```python
from build123d import *

# Parameters (mm, degrees)
SKETCH1_W           = 80
SKETCH1_H           = 100
BOSS_EXTRUDE1_DEPTH = 5
SKETCH2_W           = 80
SKETCH2_H           = 5
BOSS_EXTRUDE2_DEPTH = 20
SKETCH3_R           = 4
CUT_EXTRUDE1_DEPTH  = 107.066017178
SKETCH4_R           = 4
CUT_EXTRUDE2_DEPTH  = 68.082039325
SKETCH5_R           = 3
CUT_EXTRUDE4_DEPTH  = 68.082039325
SKETCH7_R           = 3
CUT_EXTRUDE5_DEPTH  = 10


with BuildPart() as part:
    # Sketch1 → Boss-Extrude1 (new body)
    with BuildSketch(Plane(origin=(0, 0, 0), x_dir=(0, 0, -1), z_dir=(1, 0, 0))):
        Rectangle(SKETCH1_W, SKETCH1_H)
    extrude(amount=BOSS_EXTRUDE1_DEPTH)

    # Sketch2 → Boss-Extrude2 (add)
    with BuildSketch(Plane(origin=(5, 0, 0), x_dir=(0, 0, -1), z_dir=(1, 0, 0))):
        with Locations((0, -47.5)):
            Rectangle(SKETCH2_W, SKETCH2_H)
    extrude(amount=BOSS_EXTRUDE2_DEPTH)

    # Sketch3 → Cut-Extrude1 (cut, through all)
    with BuildSketch(Plane(origin=(0, -45, 0), x_dir=(1, 0, 0), z_dir=(0, 1, 0))):
        with Locations(Location((14, 25, 0), (0, 0, 270))):
            Circle(SKETCH3_R)
        with Locations(Location((14, -25, 0), (0, 0, 270))):
            Circle(SKETCH3_R)
    extrude(amount=-CUT_EXTRUDE1_DEPTH, mode=Mode.SUBTRACT)

    # Sketch4 → Cut-Extrude2 (cut, through all)
    with BuildSketch(Plane(origin=(5, 0, 0), x_dir=(0, 0, -1), z_dir=(1, 0, 0))):
        with Locations((3, -18)):
            Circle(SKETCH4_R)
    extrude(amount=-CUT_EXTRUDE2_DEPTH, mode=Mode.SUBTRACT)

    # Sketch5 → Cut-Extrude4 (cut, through all)
    with BuildSketch(Plane(origin=(5, 0, 0), x_dir=(0, 0, -1), z_dir=(1, 0, 0))):
        with BuildLine():
            Line((-40, 50), (-40, 0))
            ThreePointArc((-40, 0), (-36.772544511, 5.320995859), (-30.562334356, 4.917565955))
            ThreePointArc((-30.562334356, 4.917565955), (-15.830972977, -2.382340063), (0.39983188, -5.001998369))
            ThreePointArc((0.39983188, -5.001998369), (28.425281663, -16.857445702), (40, -45))
            Line((40, -45), (40, 50))
            Line((40, 50), (-40, 50))
        make_face()
        with Locations((-34, 0)):
            Circle(SKETCH5_R)
    extrude(amount=-CUT_EXTRUDE4_DEPTH, mode=Mode.SUBTRACT)

    # Sketch7 → Cut-Extrude5 (cut)
    with BuildSketch(Plane.ZY):
        with Locations((-18, -25)):
            Circle(SKETCH7_R)
    extrude(amount=-CUT_EXTRUDE5_DEPTH, mode=Mode.SUBTRACT)


solid = part.part
```
Build history of the part. All positions in model axes, mm. A direction names the side the tool comes from. Coordinates: 2 decimals unless noted, no trailing zeros. Order: outer loops, then holes, each group sorted by start corner. A loop starts at its lowest first (then second) coordinate and runs counter-clockwise, first axis right, second up.
Item 1: Mould opens along Y. For faces 3 (the cylindrical face through (2.54, -2.31, 16.05)), 4 (the cylindrical face through (2.535, -14.627, -5.15)), 5 (the cylindrical face through (16.7, -47.46, 22.05)) say: released by +Y, released by -Y, zero draft, split by the parting line, or undercut.
Filled in:
face 3: released by +Y
face 4: undercut
face 5: zero draft
Item 2: Saw through at D-D on x = 21.75. List the corners of the cut face in (y, z), then the cut area to 3 significant figures.
Filled in:
outline: (-50, -40) - (-45, -40) - (-45, 40) - (-50, 40) - close
area: 400 mm2
Item 3: Drill centre lines: L1, parallel to Y at x = 1.1, z = 34; L2, parallel to X at y = -48.35, z = 25; L3, parallel to X at y = -40, z = -2. Where is each one in solid material? Low to high.
Filled in:
L1: y = -50 to -3, 3 to 6
L2: x = 0 to 10, 18 to 25
L3: x = 0 to 5
Item 4: Drop flat-ended pins along their axis: pin 1 Ø13 at (x, z) = (14, 25) entering from +Y; pin 2 Ø8 at (x, y) = (5.5, -34) entering from -Z; pin 3 Ø5 at (y, z) = (-33.5, -17.5) entering from +X. Give the stop position or say it passes through.
Filled in:
pin 1: stops at y = -45
pin 2: stops at z = -39.38
pin 3: stops at x = 5
Item 5: Saw through at A-A on z = 34. List the corners of the cut face in (x, y).
Filled in:
outline: (0, -50) - (25, -50) - (25, -45) - (5, -45) - (5, -3) - (0, -3) - close; (0, 3) - (5, 3) - (5, 6) - (0, 6) - close
Item 6: Saw through at C-C on y = -18. List the corners of the cut face in (x, z), then the cut area to 3 significant figures.
Filled in:
outline: (0, -29.51) - (5, -29.51) - (5, -7) - (0, -7) - close; (0, 1) - (5, 1) - (5, 40) - (0, 40) - close
area: 308 mm2
Item 7: Tool access for faces 1 (the flat face through (5, -25, 9)), 2 (the cylindrical face through (3, 0, 37)): list every direction of +Z, -Z, +X, -X, +Y, -Y with a clear straight run to the whole face (end or side of a thin tool).
Filled in:
face 1: +Z, -Z, +X, +Y
face 2: +X, -X
Item 8: Saw through at B-B on x = 14. List the corners of the cut face in (y, z), then the cut area to 3 significant figures.
Filled in:
outline: (-50, -40) - (-45, -40) - (-45, -29) - (-50, -29) - close; (-50, -21) - (-45, -21) - (-45, 21) - (-50, 21) - close; (-50, 29) - (-45, 29) - (-45, 40) - (-50, 40) - close
area: 320 mm2
